Verification items for the finished model (mm, model axes). A direction names the side the tool comes from. Give positions to 0.01 mm unless a question says otherwise; leave off trailing zeros. Loops run counter-clockwise (first coordinate to the right, second up) from the corner with the lowest first, then second, coordinate; pieces in that order, holes last. Notation, with made-up numbers: (84, -32) - (98, -32) arc R10 cw to (98, -25) - close; hole circle Ø11 at (80.5, 54). An arc over 180 degrees is marked (long way). Use one line per item in the form item = value.
```python
from build123d import *

# Parameters (mm, degrees)
BOSS_EXTRUDE1_DEPTH = 5
SKETCH2_R           = 4
CUT_EXTRUDE1_DEPTH  = 5


with BuildPart() as part:
    # Sketch1 → Boss-Extrude1 (new body)
    with BuildSketch(Plane.XY):
        with BuildLine():
            Line((-10, -7.5), (10, -7.5))
            ThreePointArc((10, -7.5), (11.858541226, -3.952847075), (12.5, 0))
            ThreePointArc((12.5, 0), (11.858541226, 3.952847075), (10, 7.5))
            Line((10, 7.5), (-10, 7.5))
            ThreePointArc((-10, 7.5), (-12.5, 0), (-10, -7.5))
        make_face()
        with BuildLine():
            ThreePointArc((10, 7.5), (0, 12.5), (-10, 7.5))
            Line((-10, 7.5), (10, 7.5))
        make_face()
        with BuildLine():
            ThreePointArc((-10, -7.5), (0, -12.5), (10, -7.5))
            Line((10, -7.5), (-10, -7.5))
        make_face()
        with BuildLine():
            Line((-26, -7.5), (-10, -7.5))
            ThreePointArc((-10, -7.5), (-12.5, 0), (-10, 7.5))
            Line((-10, 7.5), (-26, 7.5))
            Line((-26, 7.5), (-26, 1.5))
            Line((-26, 1.5), (-21, 1.5))
            Line((-21, 1.5), (-21, 3))
            ThreePointArc((-21, 3), (-20, 4), (-19, 3))
            Line((-19, 3), (-19, 1.5))
            Line((-19, 1.5), (-14, 1.5))
            Line((-14, 1.5), (-14, -1.5))
            Line((-14, -1.5), (-19, -1.5))
            Line((-19, -1.5), (-19, -3))
            ThreePointArc((-19, -3), (-20, -4), (-21, -3))
            Line((-21, -3), (-21, -1.5))
            Line((-21, -1.5), (-26, -1.5))
            Line((-26, -1.5), (-26, -7.5))
        make_face()
        with BuildLine():
            Line((10, -7.5), (26, -7.5))
            Line((26, -7.5), (26, -1.5))
            Line((26, -1.5), (21, -1.5))
            Line((21, -1.5), (21, -3))
            ThreePointArc((21, -3), (20, -4), (19, -3))
            Line((19, -3), (19, -1.5))
            Line((19, -1.5), (14, -1.5))
            Line((14, -1.5), (14, 1.5))
            Line((14, 1.5), (19, 1.5))
            Line((19, 1.5), (19, 3))
            ThreePointArc((19, 3), (20, 4), (21, 3))
            Line((21, 3), (21, 1.5))
            Line((21, 1.5), (26, 1.5))
            Line((26, 1.5), (26, 7.5))
            Line((26, 7.5), (10, 7.5))
            ThreePointArc((10, 7.5), (11.858541226, 3.952847075), (12.5, 0))
            ThreePointArc((12.5, 0), (11.858541226, -3.952847075), (10, -7.5))
        make_face()
    extrude(amount=BOSS_EXTRUDE1_DEPTH)

    # Sketch2 → Cut-Extrude1 (cut)
    with BuildSketch(Plane.XY.offset(5)):
        Circle(SKETCH2_R)
    extrude(amount=-CUT_EXTRUDE1_DEPTH, mode=Mode.SUBTRACT)


solid = part.part
```
1. Draft check along Y on faces 4 (the flat face through (-18, -7.5, 2)), 5 (the flat face through (21, -2, 2)), 6 (the flat face through (-26, -4, 2)). Enter one of: released by +Y, released by -Y, zero draft, split by the parting line, or undercut.
Result set:
face_4 = released by -Y
face_5 = undercut
face_6 = zero draft
2. Section check D-D, the plane y = 2.5. Record the cut outline in (x, z).
Result set:
outline = (-26, 0) - (-21, 0) - (-21, 5) - (-26, 5) - close; (-19, 0) - (-3.12, 0) - (-3.12, 5) - (-19, 5) - close; (3.12, 0) - (19, 0) - (19, 5) - (3.12, 5) - close; (21, 0) - (26, 0) - (26, 5) - (21, 5) - close
3. Scan lines: probe 1 along Y at (x, z) = (-17, 4.05); probe 2 along Y at (x, z) = (0, 1.2); probe 3 along X at (y, z) = (0.25, 3). Record each from-to range of solid material in increasing order.
Result set:
probe_1 = -7.5 to -1.5, 1.5 to 7.5
probe_2 = -12.5 to -4, 4 to 12.5
probe_3 = -14 to -3.99, 3.99 to 14
4. Tool access check on faces 1 (the flat face through (17, -1.5, 2)), 2 (the flat face through (-16, -1.5, 2)), 3 (the cylindrical face through (20, 4, 2)). Record the directions out of +Z, -Z, +X, -X, +Y, -Y that give a thin tool (end or side, any length) a straight path to the whole face; none if there is none.
Result set:
face_1 = +Z, -Z, +X
face_2 = +Z, -Z, -X
face_3 = +Z, -Z
5. Section check A-A, the plane y = 0. Record the cut outline in (x, z).
Result set:
outline = (-14, 0) - (-4, 0) - (-4, 5) - (-14, 5) - close; (4, 0) - (14, 0) - (14, 5) - (4, 5) - close
6. Depth check by flat-ended pin: pin 1 Ø1.5 at (x, z) = (24, 1.5) entering from +Y; pin 2 Ø2 at (x, z) = (7.5, 2.5) entering from +Y; pin 3 Ø2.5 at (x, z) = (20.5, 3) entering from -Y. Enter the tip coordinate at first touch or a pass-through.
Result set:
pin_1 = 7.5
pin_2 = 10.68
pin_3 = -7.5
7. Section check C-C, the plane x = 0. Record the cut outline in (y, z).
Result set:
outline = (-12.5, 0) - (-4, 0) - (-4, 5) - (-12.5, 5) - close; (4, 0) - (12.5, 0) - (12.5, 5) - (4, 5) - close
